Check sheet for the modelled part. Datum: model origin and axes. Units: mm. A direction names the side the tool comes from. Round coordinates to 2 decimals unless told otherwise and drop trailing zeros. Loops run counter-clockwise (first coordinate to the right, second up) from the corner with the lowest first, then second, coordinate; pieces in that order, holes last. Notation, with made-up numbers: M -27.75,72 L 17.25,72 A26 cw 17.25,95 Z; hole C 9.25,-13.75 d4. An arc over 180 degrees is marked long. Write item = value, one per line. Start each with the question number.
(1) Set-up check for faces 1 (the face through (19.27, 8.25, -9.97)), 2 (the face through (19.42, 2.89, 10.65)), 3 (the face through (36, 0, 0)), 4 (the face through (19.272, -4.508, -12.123)): record each of +Z, -Z, +X, -X, +Y, -Y from which the full face is reachable in a straight line by a thin tool's end or side.
(2) Cross-section at A-A on x = 27. Record the boundary of the cut face in (y, z).
(3) Go/stop test with flat-tipped pins: P1, Ø5, axis at x = 5.5, y = 5.5, coming from the +Z side; P2, Ø4, axis at x = 4.5, y = 6.5, coming from the -Z side; P3, Ø8, axis at x = 29.5, y = -9, coming from the -Z side. Record where each tip stops, or that it passes through.
(4) Cross-section at B-B on x = 2. Record the boundary of the cut face in (y, z).
(5) Scan lines: L1, parallel to Z at x = 10.9, y = 0; L2, parallel to Z at x = -4, y = 1.5. Record each from-to range of solid material in increasing order. Write a range as from..to.
from build123d import *

# Parameters (mm, degrees)
ENL_V_MAT_EXTRU_1_DEPTH      = 1.5
R_P_TITION_CIRCULAIRE1_COUNT = 6


with BuildPart() as part:
    # Esquisse1 → Base-Révolution (revolve)
    with BuildSketch(Plane.XY):
        with BuildLine():
            Line((0, 17), (14, 17))
            Line((14, 17), (16.14222201, 15.5))
            Line((16.14222201, 15.5), (19.5, 15.5))
            Line((19.5, 15.5), (20, 15))
            Line((20, 15), (20, 6))
            Line((20, 6), (35, 6))
            Line((35, 6), (36, 5))
            Line((36, 5), (36, 0))
            Line((36, 0), (16, 0))
            Line((16, 0), (11.958548116, 7))
            Line((11.958548116, 7), (9.746794345, 7))
            ThreePointArc((9.746794345, 7), (2.013063522, 11.829944009), (-6.882917236, 9.829824531))
            Line((-6.882917236, 9.829824531), (-9.750799418, 13.925584753))
            ThreePointArc((-9.750799418, 13.925584753), (-5.111998592, 16.213188163), (0, 17))
        make_face()
    revolve(axis=Axis((94.383348317, 0, 0), (-1, 0, 0)))

    # Esquisse3 → Enlèv. mat.-Extru.1 (cut)
    with BuildSketch(Plane(origin=(19.396926208, -3.420201433, 0), x_dir=(0, 0, -1), z_dir=(0.9848077530122081, -0.1736481776669306, 0))):
        with BuildLine():
            Line((-11, 3.472963553), (-18.209947962, 3.472963553))
            ThreePointArc((-18.209947962, 3.472963553), (-15.606207956, 12.856378604), (-8.539576778, 19.556428144))
            Line((-8.539576778, 19.556428144), (-5.158463097, 13.188428466))
            ThreePointArc((-5.158463097, 13.188428466), (-9.42717068, 9.141160177), (-11, 3.472963553))
        make_face()
    enl_v_mat_extru_1 = extrude(amount=-ENL_V_MAT_EXTRU_1_DEPTH, mode=Mode.SUBTRACT)

    # Répétition circulaire1: Enlèv. mat.-Extru.1 ×6 about axis
    r_p_tition_circulaire1_axis = Axis((94.383348317, 0, 0), (-1, 0, 0))
    for i in range(1, R_P_TITION_CIRCULAIRE1_COUNT):
        add(enl_v_mat_extru_1.rotate(r_p_tition_circulaire1_axis, i * 360 / R_P_TITION_CIRCULAIRE1_COUNT), mode=Mode.SUBTRACT)


solid = part.part
Result:
q1.face_1 = +X
q1.face_2 = +Z, +X
q1.face_3 = +Z, -Z, +X, +Y, -Y
q1.face_4 = -Z, +X
q2.outline = C 0,0 d12
q3.P1 = 16.73
q3.P2 = -16.39
q3.P3 = -3.32
q4.outline = C 0,0 d34; hole C 0,0 d23.66
q5.L1 = -17..-7, 7..17
q5.L2 = -16.45..-11.21, 11.21..16.45
